from build123d import *

# Parameters (mm, degrees)
SKETCH1_W           = 40
SKETCH1_H           = 40
BOSS_EXTRUDE1_DEPTH = 40
SKETCH2_W           = 10
SKETCH2_H           = 20
CUT_EXTRUDE1_DEPTH  = 40
CUT_EXTRUDE3_DEPTH  = 20


with BuildPart() as part:
    # Sketch1 → Boss-Extrude1 (new body)
    with BuildSketch(Plane.XY):
        with Locations((20, 20)):
            Rectangle(SKETCH1_W, SKETCH1_H)
    extrude(amount=BOSS_EXTRUDE1_DEPTH)

    # Sketch2 → Cut-Extrude1 (cut)
    with BuildSketch(Plane.XY.offset(40)):
        with Locations((5, 30)):
            Rectangle(SKETCH2_W, SKETCH2_H)
    extrude(amount=-CUT_EXTRUDE1_DEPTH, mode=Mode.SUBTRACT)

    # Sketch3 → Cut-Extrude3 (cut)
    with BuildSketch(Plane(origin=(0, 40, 0), x_dir=(1, 0, 0), z_dir=(0, 1, 0))):
        Polygon((40, -30), (10, 0), (10, -40), (40, -40), align=None)
    extrude(amount=-CUT_EXTRUDE3_DEPTH, mode=Mode.SUBTRACT)


solid = part.part
Source: CAD feature listing. Evaluate the final solid. Frame: model axes, mm. A direction names the side the tool comes from. Round coordinates to 2 decimals unless told otherwise and drop trailing zeros. Loops run counter-clockwise (first coordinate to the right, second up) from the corner with the lowest first, then second, coordinate; pieces in that order, holes last. Notation, with made-up numbers: M -34,86.5 L 16,86.5 A23 cw 16,119.5 Z; hole C 82.5,28 d9. An arc over 180 degrees is marked long. Return JSON: item names as keys, results as strings. Group by question number.
1. Pin query (flat end, axial travel): pin 1 (12 mm diameter, centred on x = 16, z = 16.5, fed in from +Y); pin 2 (1 mm diameter, centred on x = 23.5, y = 31.5, fed in from +Z); pin 3 (2 mm diameter, centred on y = 33, z = 20.5, fed in from -X). Return the tip coordinate at first contact, or that it passes through.
2. Material intervals for line 1 along Y through (x, z) = (16, 26); line 2 along Z through (x, y) = (14.5, 28); line 3 along Z through (x, y) = (27.5, 24.5), sorted ascending. Write a range as from..to.
3. Reachability of faces 1 (the face through (0, 10, 20)), 2 (the face through (25, 30, 15)) from +Z, -Z, +X, -X, +Y, -Y: full face, straight path, thin tool, end or side. Return the list, or none.
4. Section query B-B on z = 20.5. Output: boundary loops of the cut face in (x, y).
5. Section query D-D on z = 35.5. Output: boundary loops of the cut face in (x, y).
6. Section query A-A on x = 15. Output: boundary loops of the cut face in (y, z), and give its area (3 significant figures).
7. Section query C-C on y = 25.5. Output: boundary loops of the cut face in (x, z).
Checks:
{
 "1": {"pin 1": "stops at y = 20", "pin 2": "stops at z = 14", "pin 3": "stops at x = 29.5"},
 "2": {"line 1": "y = 0..20", "line 2": "z = 0..4.5", "line 3": "z = 0..17.5"},
 "3": {"face 1": "+Z, -Z, -X, +Y, -Y", "face 2": "+Z, -X, +Y"},
 "4": {"outline": "M 0,0 L 40,0 L 40,40 L 30.5,40 L 30.5,20 L 0,20 Z"},
 "5": {"outline": "M 0,0 L 40,0 L 40,20 L 0,20 Z"},
 "6": {"outline": "M 0,0 L 40,0 L 40,5 L 20,5 L 20,40 L 0,40 Z", "area": "900 mm²"},
 "7": {"outline": "M 10,0 L 40,0 L 40,30 Z"}
}
